from build123d import *

# Parameters (mm, degrees)
F2_R     = 7.5
F3_DEPTH = 50
F5_DEPTH = 25


with BuildPart() as f1:
    # F0 (on Front) → F1 (revolve)
    with BuildSketch(Plane.XZ):
        Polygon((-20, 30), (-10, 0), (0, 0), (0, 40), (-23.333333, 40), align=None)
    revolve(axis=Axis((0, 0, 20), (0, 0, -1)))

    # F2 (on Top) → F3 (cut)
    with BuildSketch(Plane.XY):
        Circle(F2_R)
    extrude(amount=F3_DEPTH, mode=Mode.SUBTRACT)

    # F4 (on Front) → F5 (cut, symmetric)
    with BuildSketch(Plane.XZ):
        with BuildLine():
            ThreePointArc((39.268938, 46.276736), (0, 57.353531), (-39.268938, 46.276736))
            ThreePointArc((-39.268938, 46.276736), (0, 36.659249), (39.268938, 46.276736))
        make_face()
    extrude(amount=F5_DEPTH, both=True, mode=Mode.SUBTRACT)


solid = f1.part
For this review, take the finished solid that the model builds, in its own axes (mm). Give positions to 0.01 mm unless a question says otherwise; leave off trailing zeros. Order: outer loops, then holes, each group sorted by start corner. A loop starts at its lowest first (then second) coordinate and runs counter-clockwise, first axis right, second up. Notation, with made-up numbers: M 17.25,20 L 37.25,20 A21 ccw 37.25,37 Z; hole C -5,64 d10. An arc over 180 degrees is marked long. Answer in a Markdown table with one row per item. Add a question column.
(1) For pin 1 (4 mm diameter, centred on y = 3.5, z = 26, fed in from +X); pin 2 (12 mm diameter, centred on y = 14, z = 35.5, fed in from -X); pin 3 (10 mm diameter, centred on y = 9.5, z = 15, fed in from +X), all flat-tipped, find the tip position at first contact; note any pin that passes through.
(2) Mouldability with a two-part tool opening along X and no side actions: class faces 1 (the face through (-4, 7, 0)), 2 (the face through (-7.493, 0.33, 18.236)) as +X half, -X half, draft (parallel to the pull), parting line (faces both ways), or undercut.
(3) Consider section A-A on z = 9. State the section outline as (x, y) points, and give its area (3 significant figures).
(4) Wall thickness on probe 1 along X at (y, z) = (0, 20.5); probe 2 along Y at (x, z) = (4.5, 17.5); probe 3 along X at (y, z) = (0, 14): over which ranges is each line inside the solid? List them lowest first. Write a range as [from, to].
Evaluation:
| question | item | result |
|---|---|---|
| 1 | pin 1 | stops at x = 19.09 |
| 1 | pin 2 | stops at x = -21.12 |
| 1 | pin 3 | stops at x = 15.04 |
| 2 | face 1 | draft |
| 2 | face 2 | undercut |
| 3 | outline | C 0,0 d26; hole C 0,0 d15 |
| 3 | area | 354 mm^2 |
| 4 | probe 1 | x = [-16.83, -7.5], [7.5, 16.83] |
| 4 | probe 2 | y = [-15.18, -6], [6, 15.18] |
| 4 | probe 3 | x = [-14.67, -7.5], [7.5, 14.67] |
